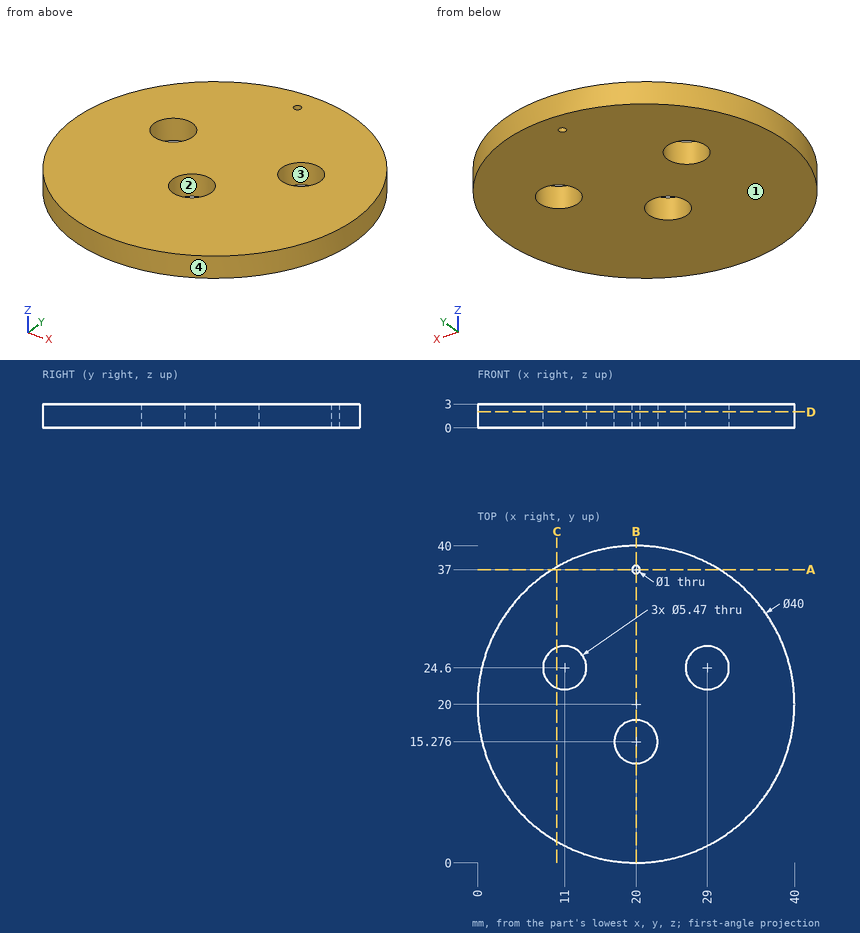
Source: three-view drawing plus pictorial views. Frame: mm from the lowest corner of the part. Coordinates: 2 decimals unless noted, no trailing zeros. Write each loop counter-clockwise with the first axis right and the second up, starting at its lowest first coordinate (ties: lowest second). Pieces come first, ordered by that corner, then holes. Notation, with made-up numbers: (48.25, 78.25) - (101.25, 78.25) arc R15 cw to (101.25, 95.25) - close; hole circle Ø4 at (-12.75, -5). An arc over 180 degrees is marked (long way). Answer as a JSON object with one key per item and string values.
Q1. First-contact query: pin 1 Ø1 at (y, z) = (27, 0.5) entering from -X (1 decimal); pin 2 Ø1.5 at (y, z) = (22, 1.5) entering from +X; pin 3 Ø1 at (y, z) = (15.5, 1) entering from +X. Flat tips, straight axial feed; report the tip coordinate or a pass-through.
Ans:
{"pin 1": "stops at x = 1.1", "pin 2": "stops at x = 39.96", "pin 3": "stops at x = 39.6"}
Q2. Section query B-B, the plane x = 20. Output: boundary loops of the cut face in (y, z).
Ans:
{"outline": "(0, 0) - (12.54, 0) - (12.54, 3) - (0, 3) - close; (18.01, 0) - (36.5, 0) - (36.5, 3) - (18.01, 3) - close; (37.5, 0) - (40, 0) - (40, 3) - (37.5, 3) - close"}
Q3. Material intervals for line 1 (Y direction, x = 20, z = 1.55); line 2 (Y direction, x = 8.5, z = 0.4) (1 decimal); line 3 (X direction, y = 37, z = 2.1) (1 decimal), sorted ascending. Write a range as [from, to].
Ans:
{"line 1": "y = [0, 12.54], [18.01, 36.5], [37.5, 40]", "line 2": "y = [3.6, 23.5], [25.7, 36.4]", "line 3": "x = [9.5, 19.5], [20.5, 30.5]"}
Q4. Section query A-A, the plane y = 37. Output: boundary loops of the cut face in (x, z) (1 decimal).
Ans:
{"outline": "(9.5, 0) - (19.5, 0) - (19.5, 3) - (9.5, 3) - close; (20.5, 0) - (30.5, 0) - (30.5, 3) - (20.5, 3) - close"}
Q5. Draft query along Y for the marked faces 1, 2, 3 and 4. Return one class per face: released by +Y, released by -Y, zero draft, split by the parting line, or undercut.
Ans:
{"face 1": "zero draft", "face 2": "undercut", "face 3": "undercut", "face 4": "split by the parting line"}
Q6. Section query D-D, the plane z = 2. Output: boundary loops of the cut face in (x, y) (1 decimal).
Ans:
{"outline": "circle Ø40 at (20, 20); hole circle Ø5.5 at (11, 24.6); hole circle Ø5.5 at (20, 15.3); hole circle Ø1 at (20, 37); hole circle Ø5.5 at (29, 24.6)"}
Q7. Section query C-C, the plane x = 10. Output: boundary loops of the cut face in (y, z) (1 decimal).
Ans:
{"outline": "(2.7, 0) - (22.1, 0) - (22.1, 3) - (2.7, 3) - close; (27.1, 0) - (37.3, 0) - (37.3, 3) - (27.1, 3) - close"}
